Check sheet for the modelled part. Datum: model origin and axes. Units: mm. A direction names the side the tool comes from. Give positions to 0.01 mm unless a question says otherwise; leave off trailing zeros. Loops run counter-clockwise (first coordinate to the right, second up) from the corner with the lowest first, then second, coordinate; pieces in that order, holes last. Notation, with made-up numbers: (86, 74.5) -> (143, 74.5) arc R14 cw to (143, 98.5) -> close; hole circle Ø1 at (63.5, 34.5). An arc over 180 degrees is marked (long way). Answer as CSV lines item,"result". Start each with the question number.
(1) Access from +Z, -Z, +X, -X, +Y, -Y to the whole of each face (thin tool, end or side, straight path). Record for faces 4 (the face through (43.75, 0, 3)), 5 (the face through (45, 0, 1)), 6 (the face through (-0.6, -27.8, 1.8)).
(2) Section check C-C on x = 31.5. Enter the section's corners in (y, z), plus the area to 3 significant figures.
(3) Gauge pin test, flat ends, axial feed: pin 1 Ø0.8 at (y, z) = (-28.5, 2.5) entering from +X; pin 2 Ø0.8 at (x, y) = (0, 28) entering from -Z; pin 3 Ø1.5 at (x, z) = (6, 3) entering from +Y; pin 4 Ø1 at (y, z) = (20, 3) entering from -X. Record the tip position at first contact, or that the pin passes through.
(4) Section check A-A on y = 10. Enter the section's corners in (x, z).
(5) Material ranges on line 1 (X direction, y = -17.5, z = 2.6); line 2 (X direction, y = -25, z = 0.3); line 3 (Y direction, x = -35, z = 1.15), recorded low to high. Write a range as from..to.
(6) Release check for a two-part mould opening along Y. For faces 1 (the face through (-1, -30, 1)), 2 (the face through (-43.75, 0, 3)), 3 (the face through (-0.6, 27.8, 1.8)) record: pulls with the +Y half, pulls with the -Y half, needs draft (parallel to the pull), parting line crosses it, or undercut.
(7) Section check B-B on x = -25.5. Enter the section's corners in (y, z).
from build123d import *

# Parameters (mm, degrees)
SKETCH_W      = 90
SKETCH_H      = 60
SKETCH_W_2    = 76
SKETCH_H_2    = 52
PAD_DEPTH     = 1
SKETCH001_W   = 90
SKETCH001_H   = 60
SKETCH001_W_2 = 85
SKETCH001_H_2 = 55.6
PAD001_DEPTH  = 1
SKETCH002_W   = 87.5
SKETCH002_H   = 57
SKETCH002_W_2 = 85
SKETCH002_H_2 = 55.6
PAD002_DEPTH  = 2
SKETCH003_W   = 5
SKETCH003_H   = 1
POCKET_DEPTH  = 58.501
CHAMFER_SIZE  = 0.4


with BuildPart() as part:
    # Sketch → Pad (new body)
    with BuildSketch(Plane.XY):
        Rectangle(SKETCH_W, SKETCH_H)
        with Locations((2, 0)):
            Rectangle(SKETCH_W_2, SKETCH_H_2, mode=Mode.SUBTRACT)
    extrude(amount=PAD_DEPTH)

    # Sketch001 → Pad001 (new body)
    with BuildSketch(Plane.XY.offset(1)):
        Rectangle(SKETCH001_W, SKETCH001_H)
        Rectangle(SKETCH001_W_2, SKETCH001_H_2, mode=Mode.SUBTRACT)
    extrude(amount=PAD001_DEPTH)

    # Sketch002 → Pad002 (new body)
    with BuildSketch(Plane.XY.offset(2)):
        Rectangle(SKETCH002_W, SKETCH002_H)
        Rectangle(SKETCH002_W_2, SKETCH002_H_2, mode=Mode.SUBTRACT)
    extrude(amount=PAD002_DEPTH)

    # Sketch003 → Pocket (cut, through all)
    with BuildSketch(Plane.XZ.offset(28.5)):
        with Locations((-30, 2.5)):
            Rectangle(SKETCH003_W, SKETCH003_H)
        with Locations((0, 2.5)):
            Rectangle(SKETCH003_W, SKETCH003_H)
        with Locations((30, 2.5)):
            Rectangle(SKETCH003_W, SKETCH003_H)
    extrude(amount=-POCKET_DEPTH, mode=Mode.SUBTRACT)

    # Chamfer
    chamfer_edges = [part.edges().sort_by_distance(p)[0] for p in [
        (0, -28.5, 4),
        (0, 28.5, 4),
    ]]
    chamfer(chamfer_edges, length=CHAMFER_SIZE)


solid = part.part
Working result:
1,face 4,"+Z, +X, +Y, -Y"
1,face 5,"+Z, -Z, +X, +Y, -Y"
1,face 6,"+Z"
2,outline,"(-30, 0) -> (-26, 0) -> (-26, 1) -> (-27.8, 1) -> (-27.8, 2) -> (-30, 2) -> close; (-28.5, 3) -> (-27.8, 3) -> (-27.8, 4) -> (-28.1, 4) -> (-28.5, 3.6) -> close; (26, 0) -> (30, 0) -> (30, 2) -> (27.8, 2) -> (27.8, 1) -> (26, 1) -> close; (27.8, 3) -> (28.5, 3) -> (28.5, 3.6) -> (28.1, 4) -> (27.8, 4) -> close"
2,area,"13.6 mm^2"
3,pin 1,"stops at x = 43.75"
3,pin 2,"stops at z = 0"
3,pin 3,"stops at y = 28.5"
3,pin 4,"stops at x = -43.75"
4,outline,"(-45, 0) -> (-36, 0) -> (-36, 1) -> (-42.5, 1) -> (-42.5, 4) -> (-43.75, 4) -> (-43.75, 2) -> (-45, 2) -> close; (40, 0) -> (45, 0) -> (45, 2) -> (43.75, 2) -> (43.75, 4) -> (42.5, 4) -> (42.5, 1) -> (40, 1) -> close"
5,line 1,"x = -43.75..-42.5, 42.5..43.75"
5,line 2,"x = -45..-36, 40..45"
5,line 3,"y = -30..-27.8, 27.8..30"
6,face 1,"pulls with the -Y half"
6,face 2,"needs draft"
6,face 3,"undercut"
7,outline,"(-30, 0) -> (-26, 0) -> (-26, 1) -> (-27.8, 1) -> (-27.8, 4) -> (-28.1, 4) -> (-28.5, 3.6) -> (-28.5, 2) -> (-30, 2) -> close; (26, 0) -> (30, 0) -> (30, 2) -> (28.5, 2) -> (28.5, 3.6) -> (28.1, 4) -> (27.8, 4) -> (27.8, 1) -> (26, 1) -> close"
